from build123d import *

# Parameters (mm, degrees)
SKETCH1_W                                            = 1212
SKETCH1_H                                            = 567
BOSS_EXTRUDE1_DEPTH                                  = 0.5
CSK_FOR_M1_6_COUNTERSUNK_FLAT_HEAD_SCREW_D           = 1.8
CSK_FOR_M1_6_COUNTERSUNK_FLAT_HEAD_SCREW_DEPTH       = 30
CSK_FOR_M1_6_COUNTERSUNK_FLAT_HEAD_SCREW_CSINK_D     = 3.6
CSK_FOR_M1_6_COUNTERSUNK_FLAT_HEAD_SCREW_CSINK_ANGLE = 90
CSK_FOR_M1_6_COUNTERSUNK_FLAT_HEAD_SCREW_TIP         = 0.540774557
SKETCH4_R                                            = 2.5
CUT_EXTRUDE1_DEPTH                                   = 3
SKETCH5_W                                            = 140
SKETCH5_H                                            = 140
CUT_EXTRUDE2_DEPTH                                   = 7


with BuildPart() as part:
    # Sketch1 → Boss-Extrude1 (new body)
    with BuildSketch(Plane(origin=(0, 0, 0), x_dir=(1, 0, 0), z_dir=(0, 1, 0))):
        with Locations((1295.999999997, 1296)):
            Rectangle(SKETCH1_W, SKETCH1_H)
    extrude(amount=BOSS_EXTRUDE1_DEPTH)

    # CSK for M1.6 Countersunk Flat Head Screw1
    with Locations(Plane(origin=(0, 0.5, 0), x_dir=(1, 0, 0), z_dir=(0, 1, 0))):
        with Locations((1899.999999997, 1577.5), (691.999999997, 1577.5), (691.999999997, 1014.5), (1899.999999997, 1014.5)):
            CounterSinkHole(CSK_FOR_M1_6_COUNTERSUNK_FLAT_HEAD_SCREW_D / 2, CSK_FOR_M1_6_COUNTERSUNK_FLAT_HEAD_SCREW_CSINK_D / 2, depth=CSK_FOR_M1_6_COUNTERSUNK_FLAT_HEAD_SCREW_DEPTH, counter_sink_angle=CSK_FOR_M1_6_COUNTERSUNK_FLAT_HEAD_SCREW_CSINK_ANGLE)
            with Locations((0, 0, -(CSK_FOR_M1_6_COUNTERSUNK_FLAT_HEAD_SCREW_DEPTH + CSK_FOR_M1_6_COUNTERSUNK_FLAT_HEAD_SCREW_TIP / 2))):  # 118° drill point
                Cone(0, CSK_FOR_M1_6_COUNTERSUNK_FLAT_HEAD_SCREW_D / 2, CSK_FOR_M1_6_COUNTERSUNK_FLAT_HEAD_SCREW_TIP, mode=Mode.SUBTRACT)

    # Sketch4 → Cut-Extrude1 (cut)
    with BuildSketch(Plane(origin=(0, 0.5, 0), x_dir=(1, 0, 0), z_dir=(0, 1, 0))):
        with Locations(Location((776.999999997, 1098.5, 0), (0, 0, 270))):
            Circle(SKETCH4_R)
        with Locations(Location((814.999999997, 1098.5, 0), (0, 0, 270))):
            Circle(SKETCH4_R)
    extrude(amount=-CUT_EXTRUDE1_DEPTH, mode=Mode.SUBTRACT)

    # Sketch5 → Cut-Extrude2 (cut)
    with BuildSketch(Plane(origin=(0, 0.5, 0), x_dir=(1, 0, 0), z_dir=(0, 1, 0))):
        with Locations((1290.243608368, 1153.58)):
            Rectangle(SKETCH5_W, SKETCH5_H)
    extrude(amount=-CUT_EXTRUDE2_DEPTH, mode=Mode.SUBTRACT)


solid = part.part
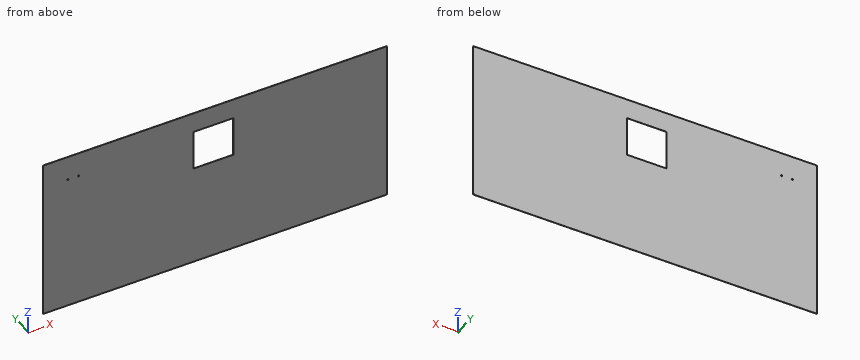
Geometry: final body of the model. Coordinates: model frame, mm. Give positions to 0.01 mm unless a question says otherwise; leave off trailing zeros. Loops run counter-clockwise (first coordinate to the right, second up) from the corner with the lowest first, then second, coordinate; pieces in that order, holes last. Notation, with made-up numbers: M 32,42.5 L 61,42.5 A23 ccw 61,69.5 Z; hole C 42.25,-23 d5. An arc over 180 degrees is marked long. Put each result on its own line as item: value. Start each with the question number.
1) Cut plane A-A (z = -1196). Output: boundary loops of the cut face in (x, y), then the cut area to 3 significant figures.
2) Ray query, line 1 along X through (y, z) = (0.35, -1098.5); line 2 along X through (y, z) = (0.1, -1182.5); line 3 along Z through (x, y) = (777, 0.25). Return the intervals inside material, ascending.
3) Cut plane B-B (y = 0.3). Output: boundary loops of the cut face in (x, z), then the cut area to 3 significant figures.
Verdict:
1. outline: M 690,0 L 1220.24,0 L 1220.24,0.5 L 690,0.5 Z; M 1360.24,0 L 1902,0 L 1902,0.5 L 1360.24,0.5 Z
1. area: 536 mm2
2. line 1: 690 to 774.5, 779.5 to 812.5, 817.5 to 1220.24, 1360.24 to 1902
2. line 2: 690 to 1220.24, 1360.24 to 1902
2. line 3: -1579.5 to -1101, -1096 to -1012.5
3. outline: M 690,-1579.5 L 1902,-1579.5 L 1902,-1012.5 L 690,-1012.5 Z; hole C 692,-1577.5 d3.2; hole C 692,-1014.5 d3.2; hole C 777,-1098.5 d5; hole C 815,-1098.5 d5; hole M 1220.24,-1223.58 L 1360.24,-1223.58 L 1360.24,-1083.58 L 1220.24,-1083.58 Z; hole C 1900,-1577.5 d3.2; hole C 1900,-1014.5 d3.2
3. area: 668,000 mm2
